from build123d import *

# Parameters (mm, degrees)
F1_DEPTH = 63.5
F0_W     = 25.4
F0_H     = 19.0246
F2_DEPTH = 25.4
F4_DEPTH = 7.9375


# Not quite as in the source:
# - a feature names something its author has since deleted; it is built from what else it names


with BuildPart() as f1:
    # F0 (on Front) → F1 (new body, symmetric)
    with BuildSketch(Plane.XZ):
        Polygon((-41.275, -9.525), (41.275, -9.525), (41.275, 9.525), (22.225, 9.525), (-41.275, 9.525), align=None)
    extrude(amount=F1_DEPTH, both=True)

    # F0 (on Front) → F2 (join, symmetric)
    with BuildSketch(Plane.XZ):
        with BuildLine():
            Line((22.225, 9.525), (41.275, 9.525))
            Line((41.275, 9.525), (41.275, 27.0002))
            ThreePointArc((41.275, 27.0002), (45.9246798487, 38.2255201513), (57.15, 42.8752))
            Line((57.15, 42.8752), (60.325, 42.8752))
            Line((60.325, 42.8752), (60.325, 61.8998))
            Line((60.325, 61.8998), (57.15, 61.8998))
            ThreePointArc((57.15, 61.8998), (32.4632742898, 51.6794835164), (22.225, 27.0002))
            Line((22.225, 27.0002), (22.225, 9.525))
        make_face()
        with Locations((73.025, 52.3875)):
            Rectangle(F0_W, F0_H)
    extrude(amount=F2_DEPTH, both=True)

    # F0 (on Front) → F3 (revolve)
    with BuildSketch(Plane.XZ):
        Polygon((85.725, 66.675), (85.725, 61.8998), (85.725, 42.8752), (85.725, 38.1), (111.125, 38.1), (111.125, 66.675), align=None)
    revolve(axis=Axis((85.725, 0, 52.3875), (0, 0, -1)))

    # F0 (on Front) → F4 (join, symmetric)
    with BuildSketch(Plane.XZ):
        with BuildLine():
            add(Edge.make_bspline(
                [(-41.275, 9.525), (-41.2365756929, 37.5034026802), (4.0239142254, 63.6744350195), (57.15, 61.8998)],
                knots=[0, 0, 0, 0, 111.4926019969, 111.4926019969, 111.4926019969, 111.4926019969], degree=3))
            Line((-41.275, 9.525), (22.225, 9.525))
            Line((22.225, 9.525), (22.225, 27.0002))
            ThreePointArc((22.225, 27.0002), (32.4632742898, 51.6794835164), (57.15, 61.8998))
        make_face()
    extrude(amount=F4_DEPTH, both=True)


solid = f1.part
Design review of the part built by this model. Coordinates are the model's own, in mm. A direction names the side the tool comes from. Give positions to 0.01 mm unless a question says otherwise; leave off trailing zeros. Order: outer loops, then holes, each group sorted by start corner. A loop starts at its lowest first (then second) coordinate and runs counter-clockwise, first axis right, second up.
1. Tool access review of faces 1 (the flat face through (46, -25.4, 42)), 2 (the flat face through (-2, -7.938, 31)), 3 (the cylindrical face through (45.8, -0.4, 38.1)): name each direction out of +Z, -Z, +X, -X, +Y, -Y from which nothing blocks a thin tool from reaching the whole face with its end or side.
Solution:
face 1: +Z, +X, -X, -Y
face 2: +Z, -X, -Y
face 3: -Z, +Y, -Y
2. Mouldability with a two-part tool opening along Z and no side actions: class faces 4 (the flat face through (41.275, -1, 4)), 5 (the cylindrical face through (32.736, 16.547, 51.949)), 6 (the flat face through (-1, -1, -9.525)) as +Z half, -Z half, draft (parallel to the pull), parting line (faces both ways), or undercut.
Solution:
face 4: draft
face 5: +Z half
face 6: -Z half
3. For pin 1 Ø8.5 at (x, y) = (67.5, 5.5) entering from -Z; pin 2 Ø15.5 at (x, z) = (12.5, 40.5) entering from +Y; pin 3 Ø2 at (y, z) = (28, 50) entering from -X; pin 4 Ø5 at (y, z) = (-18, 16) entering from -X (3 decimals), all flat-tipped, find the tip position at first contact; note any pin that passes through.
Solution:
pin 1: stops at z = 38.1
pin 2: stops at y = 7.94
pin 3: passes through
pin 4: stops at x = 22.225
4. Add section B-B, the plane z = -3.5. State the section outline as (x, y) points (3 decimals), then the cut area to 3 significant figures.
Solution:
outline: (-41.275, -63.5) - (41.275, -63.5) - (41.275, 63.5) - (-41.275, 63.5) - close
area: 10,500 mm2
5. Add section A-A, the plane y = 47. State the section outline as (x, z) points (3 decimals).
Solution:
outline: (-41.275, -9.525) - (41.275, -9.525) - (41.275, 9.525) - (-41.275, 9.525) - close
6. Add section C-C, the plane y = 22. State the section outline as (x, z) points (3 decimals).
Solution:
outline: (-41.275, -9.525) - (41.275, -9.525) - (41.275, 27) arc R15.875 cw to (57.15, 42.875) - (73.03, 42.875) - (73.03, 38.1) - (98.42, 38.1) - (98.42, 66.675) - (73.03, 66.675) - (73.03, 61.9) - (57.15, 61.9) arc R34.925 ccw to (22.225, 27) - (22.225, 9.525) - (-41.275, 9.525) - close
7. To check wall thickness, follow L1, parallel to Y at x = 9.5, z = 38.5; L2, parallel to Z at x = 6.5, y = 41.5 (3 decimals); L3, parallel to Y at x = 41.5, z = 41. State the ranges of each line that lie inside material, in increasing order.
Solution:
L1: y = -7.94 to 7.94
L2: z = -9.525 to 9.525
L3: y = -25.4 to 25.4
